Read the model definition and answer for the solid it produces. Units are mm, in the model's axes. A direction names the side the tool comes from. Round coordinates to 2 decimals unless told otherwise and drop trailing zeros. Order: outer loops, then holes, each group sorted by start corner. A loop starts at its lowest first (then second) coordinate and runs counter-clockwise, first axis right, second up. Notation, with made-up numbers: (4.25, 20) -> (62.25, 20) arc R15 cw to (62.25, 25) -> close; hole circle Ø4 at (22.25, -10). An arc over 180 degrees is marked (long way). One line per item, written item: value. Start each with the question number.
1. Section D-D (x = -9) is taken. Give the vertices of the cut face in (y, z), then the cut area to 3 significant figures.
2. For faces 5 (the face through (0, -4.027, 5)), 6 (the face through (8, 0, 3)), 7 (the face through (-3.2, -3, 7)), determine the directions among +Z, -Z, +X, -X, +Y, -Y from which every point of the face is accessible in a straight line to the end or side of a thin tool.
3. Consider line 1 (X direction, y = -5, z = 4.5); line 2 (X direction, y = 6, z = 4.25); line 3 (Y direction, x = 0, z = 0.95). Determine where each line is inside the solid, lowest interval first.
4. Section C-C (y = 13) is taken. Give the vertices of the cut face in (x, z).
5. Section B-B (x = 0) is taken. Give the vertices of the cut face in (y, z).
6. The mould has two halves that part along Z. Classify faces 1 (the face through (16.7, -0.3, 5.7)), 2 (the face through (19, 0, 8)), 3 (the face through (-16.7, -0.3, 5.7)), 4 (the face through (3.5, 1.99, 5.03)): released by +Z, released by -Z, zero draft, split by the parting line, or undercut.
7. Flat-ended cylindrical pins translate along their axes: pin 1 Ø2 at (x, y) = (17, -3.5) entering from -Z; pin 2 Ø7 at (x, y) = (-2.5, 2.5) entering from +Z; pin 3 Ø2 at (x, z) = (-1, 5) entering from -Y; pin 4 Ø4.5 at (x, y) = (0, 0) entering from -Z. Find the tip coordinate at first contact, or state that the pin passes through.
8. Section A-A (z = 6.5) is taken. Give the vertices of the cut face in (x, y) (3 decimals).
from build123d import *

# Parameters (mm, degrees)
F0_W     = 45
F0_H     = 37
F1_DEPTH = 8
F3_DEPTH = 37.001
F5_R     = 7
F6_DEPTH = 4
F4_R     = 2.75
F7_DEPTH = 25
F9_DEPTH = 4


with BuildPart() as f1:
    # F0 (on Top) → F1 (new body)
    with BuildSketch(Plane.XY):
        Rectangle(F0_W, F0_H)
    extrude(amount=F1_DEPTH)

    # F2 (on face) → F3 (cut, through all)
    with BuildSketch(Plane.XZ.offset(18.5)):
        Polygon((15.7, 8), (-15.7, 8), (-17.7, 3.392867), (-17.7, 3), (17.7, 3), (17.7, 3.392867), align=None)
    extrude(amount=-F3_DEPTH, mode=Mode.SUBTRACT)

    # F5 (on face) → F6 (join)
    with BuildSketch(Plane.XY.offset(3)):
        Circle(F5_R)
    extrude(amount=F6_DEPTH)

    # F4 (on face) → F7 (cut)
    with BuildSketch(Plane(origin=(0, 0, 0), x_dir=(1, 0, 0), z_dir=(0, 0, -1))):
        Circle(F4_R)
    extrude(amount=-F7_DEPTH, mode=Mode.SUBTRACT)

    # F8 (on face) → F9 (cut)
    with BuildSketch(Plane.XY.offset(7)):
        Polygon((2.325, -4.027018), (4.65, 0), (2.325, 4.027018), (-2.325, 4.027018), (-4.65, 0), (-2.325, -4.027018), align=None)
    extrude(amount=-F9_DEPTH, mode=Mode.SUBTRACT)


solid = f1.part
Answer:
1. outline: (-18.5, 0) -> (18.5, 0) -> (18.5, 3) -> (-18.5, 3) -> close
1. area: 111 mm^2
2. face 5: +Z
2. face 6: none
2. face 7: +Z, +Y, -Y
3. line 1: -22.5 to -17.22, -4.9 to 4.9, 17.22 to 22.5
3. line 2: -22.5 to -17.33, -3.61 to 3.61, 17.33 to 22.5
3. line 3: -18.5 to -2.75, 2.75 to 18.5
4. outline: (-22.5, 0) -> (22.5, 0) -> (22.5, 8) -> (15.7, 8) -> (17.7, 3.39) -> (17.7, 3) -> (-17.7, 3) -> (-17.7, 3.39) -> (-15.7, 8) -> (-22.5, 8) -> close
5. outline: (-18.5, 0) -> (-2.75, 0) -> (-2.75, 3) -> (-4.03, 3) -> (-4.03, 7) -> (-7, 7) -> (-7, 3) -> (-18.5, 3) -> close; (2.75, 0) -> (18.5, 0) -> (18.5, 3) -> (7, 3) -> (7, 7) -> (4.03, 7) -> (4.03, 3) -> (2.75, 3) -> close
6. face 1: undercut
6. face 2: released by +Z
6. face 3: undercut
6. face 4: zero draft
7. pin 1: z = 0
7. pin 2: z = 7
7. pin 3: y = -7
7. pin 4: through
8. outline: (-22.5, -18.5) -> (-16.351, -18.5) -> (-16.351, 18.5) -> (-22.5, 18.5) -> close; circle Ø14 at (0, 0); (16.351, -18.5) -> (22.5, -18.5) -> (22.5, 18.5) -> (16.351, 18.5) -> close; hole (-4.65, 0) -> (-2.325, -4.027) -> (2.325, -4.027) -> (4.65, 0) -> (2.325, 4.027) -> (-2.325, 4.027) -> close
